Job drawing, mm, ordinate dimensions from the low corner. One solid piece. Give positions to 0.01 mm unless a question says otherwise; leave off trailing zeros. Loops run counter-clockwise (first coordinate to the right, second up) from the corner with the lowest first, then second, coordinate; pieces in that order, holes last. Notation, with made-up numbers: M 69,28.5 L 83,28.5 A7 ccw 83,34.5 Z; hole C 26,59.25 d9. An arc over 180 degrees is marked long. Answer as CSV lines item,"result".
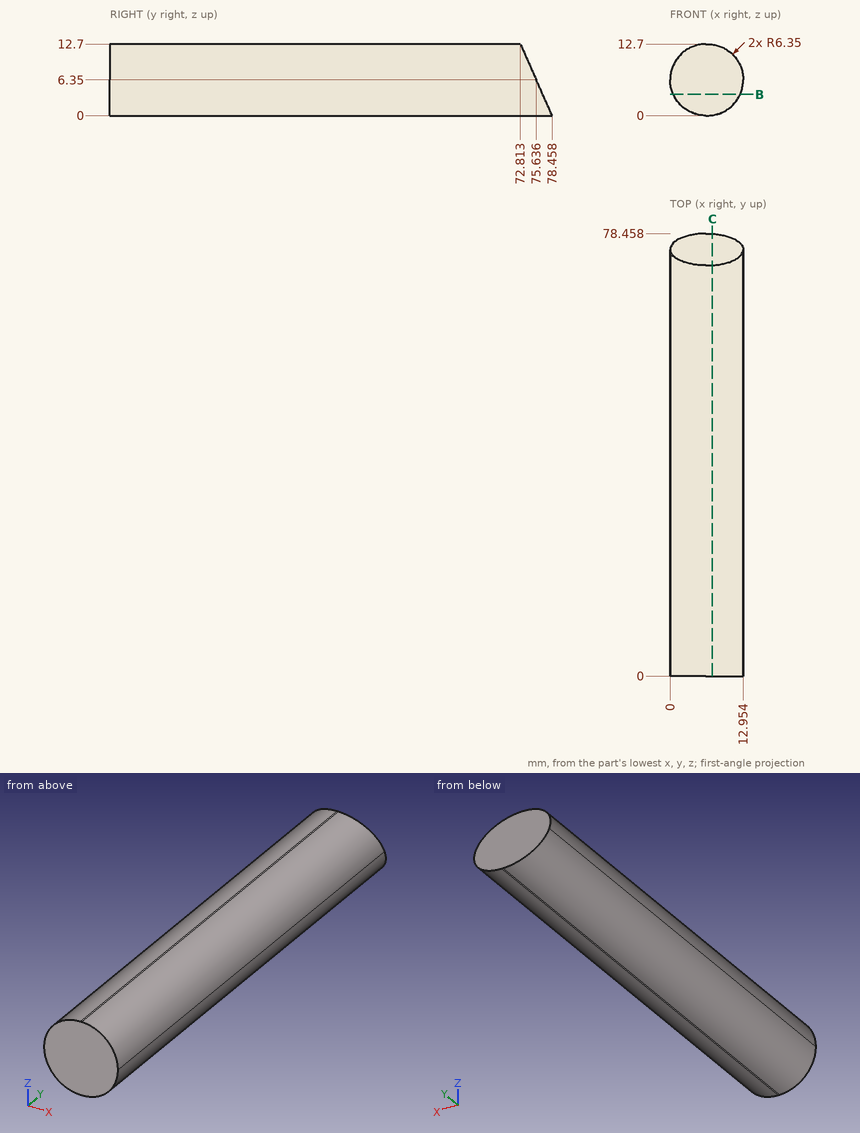
1) Band-saw the part on C-C on x = 7.5. Give the cut face in (y, z).
Answer below:
outline,"M 0,0.06 L 78.43,0.06 L 72.84,12.64 L 0,12.64 Z"
2) Band-saw the part on B-B on z = 3.75. Give the cut face in (x, y), and give its area (3 significant figures).
Answer below:
outline,"M 0.56,0 L 12.4,0 L 12.4,76.79 L 0.56,76.79 Z"
area,"909 mm^2"
3) Drill centre lines: line 1 (Z direction, x = 6.25, y = 36); line 2 (X direction, y = 27, z = 6) (1 decimal); line 3 (Y direction, x = 3.75, z = 11.75) (1 decimal). Where is each one in solid material? Low to high. Write a range as from..to.
Answer below:
line 1,"z = 0..12.7"
line 2,"x = 0..12.9"
line 3,"y = 0..73.2"
4) Flat gauge pins, fed straight in: pin 1 (1.5 mm diameter, centred on x = 8, z = 3, fed in from +Y); pin 2 (5 mm diameter, centred on y = 57, z = 3.5, fed in from +X); pin 3 (1.5 mm diameter, centred on y = 9.5, z = 8.5, fed in from +X). Where does each tip first touch, or does it go through?
Answer below:
pin 1,"stops at y = 77.46"
pin 2,"stops at x = 12.94"
pin 3,"stops at x = 12.8"
